Verification items for the finished model (mm, model axes). A direction names the side the tool comes from. Give positions to 0.01 mm unless a question says otherwise; leave off trailing zeros. Order: outer loops, then holes, each group sorted by start corner. A loop starts at its lowest first (then second) coordinate and runs counter-clockwise, first axis right, second up. Notation, with made-up numbers: (-13.5, 88) - (23.5, 88) arc R16 ccw to (23.5, 93) - close; hole circle Ø6 at (37.25, -15.5). An arc over 180 degrees is marked (long way). Answer as a JSON object with one key per item and string values. Group by question number.
(1) Section check A-A (x = 0). Record the boundary of the cut face in (y, z) (3 decimals).
(2) Access from +Z, -Z, +X, -X, +Y, -Y to the whole of each face (thin tool, end or side, straight path). Record for faces 1 (the face through (34.2, 68, 17.8)), 2 (the face through (-36.156, 1.521, 19.414)), 3 (the face through (0.12, 72.93, -44.006)), 4 (the face through (35.32, 73.07, 18.53)), 5 (the face through (-17, 78, -31)).
(3) Section check B-B (z = 0). Record the boundary of the cut face in (x, y).
(4) Thickness scan on line 1 (X direction, y = 30, z = 0); line 2 (Y direction, x = -2, z = 41); line 3 (X direction, y = 73.5, z = 22.5). Record the ranges inside material, lowest first.
(5) Depth check by flat-ended pin: pin 1 Ø6 at (x, y) = (-9.5, 40.5) entering from -Z; pin 2 Ø12 at (x, y) = (0.5, 29.5) entering from -Z; pin 3 Ø5 at (y, z) = (27.5, -13) entering from +X. Enter the tip coordinate at first touch or a pass-through.
(6) Mould release check, pull along X, two halves, no side actions. Record for faces 6 (the face through (11.009, 40.989, 34.958)), 7 (the face through (0.451, 1.521, -40.394)), 8 (the face through (-33.123, 3, -20.21)): +X half, -X half, draft (parallel to the pull), parting line (faces both ways), or undercut.
```python
from build123d import *

# Parameters (mm, degrees)
SKETCH3_R           = 45
SKETCH3_R_2         = 35.15
BOSS_EXTRUDE4_DEPTH = 3
SKETCH4_R           = 36.65
SKETCH4_R_2         = 35.15
BOSS_EXTRUDE5_DEPTH = 75
FILLET1_R           = 2
SKETCH7_R           = 1.5
CUT_EXTRUDE2_DEPTH  = 99.361577865
BOSS_EXTRUDE7_START = -10
BOSS_EXTRUDE7_DEPTH = 10
SKETCH9_R           = 1.65
CUT_EXTRUDE3_DEPTH  = 10
FILLET2_R           = 3


with BuildPart() as part:
    # Sketch3 → Boss-Extrude4 (new body)
    with BuildSketch(Plane(origin=(0, 0, 0), x_dir=(1, 0, 0), z_dir=(0, 1, 0))):
        with Locations(Location((0, 0, 0), (0, 0, 270))):
            Circle(SKETCH3_R)
        with Locations(Location((0, 0, 0), (0, 0, 270))):
            Circle(SKETCH3_R_2, mode=Mode.SUBTRACT)
    extrude(amount=BOSS_EXTRUDE4_DEPTH)

    # Sketch4 → Boss-Extrude5 (add)
    with BuildSketch(Plane(origin=(0, 3, 0), x_dir=(1, 0, 0), z_dir=(0, 1, 0))):
        with Locations(Location((0, 0, 0), (0, 0, 270))):
            Circle(SKETCH4_R)
        with Locations(Location((0, 0, 0), (0, 0, 270))):
            Circle(SKETCH4_R_2, mode=Mode.SUBTRACT)
    extrude(amount=BOSS_EXTRUDE5_DEPTH)

    # Fillet1
    fillet1_edges = [part.edges().sort_by_distance(p)[0] for p in [
        (0, 3, -36.65),
    ]]
    fillet(fillet1_edges, radius=FILLET1_R)

    # Sketch7 → Cut-Extrude2 (cut, through all)
    with BuildSketch(Plane(origin=(0, 3, 0), x_dir=(1, 0, 0), z_dir=(0, 1, 0))):
        with Locations(Location((0, 41.825, 0), (0, 0, 270))):
            Circle(SKETCH7_R)
        with Locations(Location((36.221512513, 20.9125, 0), (0, 0, 270))):
            Circle(SKETCH7_R)
        with Locations(Location((36.221512513, -20.9125, 0), (0, 0, 270))):
            Circle(SKETCH7_R)
        with Locations(Location((0, -41.825, 0), (0, 0, 270))):
            Circle(SKETCH7_R)
        with Locations(Location((-36.221512513, -20.9125, 0), (0, 0, 270))):
            Circle(SKETCH7_R)
        with Locations(Location((-36.221512513, 20.9125, 0), (0, 0, 270))):
            Circle(SKETCH7_R)
    extrude(amount=-CUT_EXTRUDE2_DEPTH, mode=Mode.SUBTRACT)

    # Sketch8 → Boss-Extrude7 (add)
    with BuildSketch(Plane(origin=(0, 78, 0), x_dir=(1, 0, 0), z_dir=(0, 1, 0)).offset(BOSS_EXTRUDE7_START)):
        with BuildLine():
            ThreePointArc((-5.10069415, 36.293324719), (0, 36.65), (5.10069415, 36.293324719))
            ThreePointArc((5.10069415, 36.293324719), (0, 44.007131423), (-5.10069415, 36.293324719))
        make_face()
        with BuildLine():
            ThreePointArc((28.88059412, -22.563993071), (38.11129376, -22.003565711), (33.98128827, -13.729331649))
            ThreePointArc((33.98128827, -13.729331649), (31.739831049, -18.325), (28.88059412, -22.563993071))
        make_face()
        with BuildLine():
            ThreePointArc((-33.98128827, -13.729331649), (-38.11129376, -22.003565711), (-28.88059412, -22.563993071))
            ThreePointArc((-28.88059412, -22.563993071), (-31.739831049, -18.325), (-33.98128827, -13.729331649))
        make_face()
    extrude(amount=BOSS_EXTRUDE7_DEPTH)

    # Sketch9 → Cut-Extrude3 (cut)
    with BuildSketch(Plane(origin=(0, 78, 0), x_dir=(1, 0, 0), z_dir=(0, 1, 0))):
        with Locations(Location((0, 39.5, 0), (0, 0, 270))):
            Circle(SKETCH9_R)
        with Locations(Location((34.208003449, -19.75, 0), (0, 0, 270))):
            Circle(SKETCH9_R)
        with Locations(Location((-34.208003449, -19.75, 0), (0, 0, 270))):
            Circle(SKETCH9_R)
    extrude(amount=-CUT_EXTRUDE3_DEPTH, mode=Mode.SUBTRACT)

    # Fillet2
    fillet2_edges = [part.edges().sort_by_distance(p)[0] for p in [
        (28.88059412, 73, 22.563993071),
        (33.98128827, 73, 13.729331649),
        (-33.98128827, 73, 13.729331649),
        (-28.88059412, 73, 22.563993071),
        (5.10069415, 73, -36.293324719),
        (-5.10069415, 73, -36.293324719),
    ]]
    fillet(fillet2_edges, radius=FILLET2_R)


solid = part.part
```
Solutions:
{
 "1": {"outline": "(0, -45) - (3, -45) - (3, -43.325) - (0, -43.325) - close; (0, -40.325) - (3, -40.325) - (3, -38.65) arc R2 cw to (5, -36.65) - (68, -36.65) - (68, -37.85) - (78, -37.85) - (78, -35.15) - (0, -35.15) - close; (0, 35.15) - (78, 35.15) - (78, 36.65) - (5, 36.65) arc R2 cw to (3, 38.65) - (3, 40.325) - (0, 40.325) - close; (0, 43.325) - (3, 43.325) - (3, 45) - (0, 45) - close; (68, -44.007) - (78, -44.007) - (78, -41.15) - (68, -41.15) - close"},
 "2": {"face 1": "+Z, +X", "face 2": "-Y", "face 3": "-Z, +Y", "face 4": "+Y", "face 5": "+Z, -Z, +X, -X, +Y"},
 "3": {"outline": "(-45, 0) - (-35.15, 0) - (-35.15, 78) - (-36.65, 78) - (-36.65, 5) arc R2 cw to (-38.65, 3) - (-45, 3) - close; (35.15, 0) - (45, 0) - (45, 3) - (38.65, 3) arc R2 cw to (36.65, 5) - (36.65, 78) - (35.15, 78) - close"},
 "4": {"line 1": "x = -36.65 to -35.15, 35.15 to 36.65", "line 2": "y = 0 to 3", "line 3": "x = -37.79 to -27.01, 27.01 to 37.79"},
 "5": {"pin 1": "stops at z = -36.07", "pin 2": "stops at z = -36.65", "pin 3": "stops at x = 35.11"},
 "6": {"face 6": "parting line", "face 7": "undercut", "face 8": "draft"}
}
